CAD build for the part. Positions are in the model's coordinates, mm. A direction names the side the tool comes from. Give positions to 0.01 mm unless a question says otherwise; leave off trailing zeros. Order: outer loops, then holes, each group sorted by start corner. A loop starts at its lowest first (then second) coordinate and runs counter-clockwise, first axis right, second up.
Item 1: Wall check: L1, parallel to X at y = -12.6, z = 22.5 (3 decimals); L2, parallel to Z at x = -20, y = -12.4 (3 decimals); L3, parallel to X at y = -11.25, z = 21.5. Give the ranges that are in metal, low to high.
Item 2: Band-saw the part on A-A on z = 7.5. Give the cut face in (x, y) (3 decimals).
Item 3: Band-saw the part on C-C on x = 1. Give the cut face in (y, z), plus the area to 3 significant figures.
Item 4: Band-saw the part on B-B on y = -11.5. Give the cut face in (x, z) (3 decimals), plus the area to 3 significant figures.
Item 5: Two-plate mould, pull along X, no slides. Class faces 1 (the flat face through (12, -8, -14)), 2 (the flat face through (-11.5, -8, -4)), 3 (the cylindrical face through (16.548, -7.888, -13.604)): released by +X, released by -X, zero draft, split by the parting line, or undercut.
Item 6: Flat gauge pins, fed straight in: P1, Ø1.1, axis at y = -11, z = -10.5, coming from the +X side; P2, Ø1.4, axis at x = 10.5, y = -4, coming from the +Z side; P3, Ø2, axis at x = -20, y = -4, coming from the -Z side; P4, Ø22.5, axis at x = -12, z = 10, coming from the +Y side. Where does each tip first touch, or does it go through?
Item 7: Band-saw the part on D-D on z = -3. Give the cut face in (x, y).
Item 8: Which spindle directions (+Z, -Z, +X, -X, +Y, -Y) get a long thin tool onto all of the face, cutting with end or side? Do faces 4 (the flat face through (0, -10, 16)), 5 (the flat face through (-24.2, -7.89, -6.13)), 6 (the cylindrical face through (7.61, -7.89, -13.1)), 7 (the flat face through (-11, -8, -7)), 8 (the flat face through (30, -11, 11)). Say none if no direction does.
```python
from build123d import *

# Parameters (mm, degrees)
F1_DEPTH       = 16
F2_W           = 20
F2_H           = 40
F3_DEPTH       = 50
F5_D           = 4.75
F5_CSINK_D     = 8
F5_CSINK_ANGLE = 90


with BuildPart() as f1:
    # F0 (on Front) → F1 (new body)
    with BuildSketch(Plane.XZ):
        with BuildLine():
            Line((-11.5, 0), (0, 0))
            Line((0, 0), (11.5, 0))
            Line((11.5, 0), (11.5, -7))
            Line((11.5, -7), (9.75, -7))
            ThreePointArc((9.75, -7), (7.6286796564, -7.8786796564), (6.75, -10))
            Line((6.75, -10), (6.75, -11))
            ThreePointArc((6.75, -11), (7.6286796564, -13.1213203436), (9.75, -14))
            Line((9.75, -14), (14.5978726692, -14))
            ThreePointArc((14.5978726692, -14), (16.5746603892, -13.5926365315), (18.2293396683, -12.4369241241))
            Line((18.2293396683, -12.4369241241), (30, 0))
            Line((30, 0), (30, 30))
            Line((30, 30), (0, 30))
            Line((0, 30), (-30, 30))
            Line((-30, 30), (-30, 0))
            Line((-30, 0), (-18.2293396683, -12.4369241241))
            ThreePointArc((-18.2293396683, -12.4369241241), (-16.5746603892, -13.5926365315), (-14.5978726692, -14))
            Line((-14.5978726692, -14), (-9.75, -14))
            ThreePointArc((-9.75, -14), (-7.6286796564, -13.1213203436), (-6.75, -11))
            Line((-6.75, -11), (-6.75, -10))
            ThreePointArc((-6.75, -10), (-7.6286796564, -7.8786796564), (-9.75, -7))
            Line((-9.75, -7), (-11.5, -7))
            Line((-11.5, -7), (-11.5, 0))
        make_face()
    extrude(amount=F1_DEPTH)

    # F2 (on Right) → F3 (cut, symmetric)
    with BuildSketch(Plane.YZ):
        with Locations((0, 22)):
            Rectangle(F2_W, F2_H)
    extrude(amount=F3_DEPTH, both=True, mode=Mode.SUBTRACT)

    # F5 (through all)
    with Locations(Plane.XZ.offset(16)):
        with Locations((20, 22.5), (20, 7.5), (-20, 22.5), (-20, 7.5)):
            CounterSinkHole(F5_D / 2, F5_CSINK_D / 2, counter_sink_angle=F5_CSINK_ANGLE)


solid = f1.part
```
The answers:
1. L1: x = -30 to -22.375, -17.625 to 17.625, 22.375 to 30
1. L2: z = -10.566 to 5.125, 9.875 to 20.125, 24.875 to 30
1. L3: x = -30 to -22.15, -17.85 to 17.85, 22.15 to 30
2. outline: (-30, -16) - (-24, -16) - (-22.375, -14.375) - (-22.375, -10) - (-30, -10) - close; (-17.625, -14.375) - (-16, -16) - (16, -16) - (17.625, -14.375) - (17.625, -10) - (-17.625, -10) - close; (22.375, -14.375) - (24, -16) - (30, -16) - (30, -10) - (22.375, -10) - close
3. outline: (-16, 0) - (0, 0) - (0, 2) - (-10, 2) - (-10, 30) - (-16, 30) - close
3. area: 200 mm2
4. outline: (-30, 0) - (-18.229, -12.437) arc R5 ccw to (-14.598, -14) - (-9.75, -14) arc R3 ccw to (-6.75, -11) - (-6.75, -10) arc R3 ccw to (-9.75, -7) - (-11.5, -7) - (-11.5, 0) - (11.5, 0) - (11.5, -7) - (9.75, -7) arc R3 ccw to (6.75, -10) - (6.75, -11) arc R3 ccw to (9.75, -14) - (14.598, -14) arc R5 ccw to (18.229, -12.437) - (30, 0) - (30, 30) - (-30, 30) - close; hole circle Ø4.75 at (-20, 7.5); hole circle Ø4.75 at (-20, 22.5); hole circle Ø4.75 at (20, 7.5); hole circle Ø4.75 at (20, 22.5)
4. area: 2,120 mm2
5. face 1: zero draft
5. face 2: undercut
5. face 3: released by +X
6. P1: stops at x = 20.58
6. P2: stops at z = 2
6. P3: stops at z = -11.62
6. P4: stops at y = 0
7. outline: (-27.16, -16) - (-11.5, -16) - (-11.5, 0) - (-27.16, 0) - close; (11.5, -16) - (27.16, -16) - (27.16, 0) - (11.5, 0) - close
8. face 4: +Z, +X, -X, +Y
8. face 5: -Z, -X, +Y, -Y
8. face 6: -Z, +Y, -Y
8. face 7: +Y, -Y
8. face 8: +Z, -Z, +X, +Y, -Y
